Geometry: final body of the model. Coordinates: model frame, mm. A direction names the side the tool comes from. Round coordinates to 2 decimals unless told otherwise and drop trailing zeros. Loops run counter-clockwise (first coordinate to the right, second up) from the corner with the lowest first, then second, coordinate; pieces in that order, holes last. Notation, with made-up numbers: (54.25, 69) - (97.25, 69) arc R16 cw to (97.25, 99) - close; hole circle Ø5 at (-10, 40.25). An arc over 180 degrees is marked (long way). Answer as CSV lines item,"result".
from build123d import *

# Parameters (mm, degrees)
F0_R     = 1.5
F2_DEPTH = 35
F1_R     = 3
F3_DEPTH = 2.52
F4_R     = 1


with BuildPart() as f2:
    # F0 (on Top) → F2 (new body)
    with BuildSketch(Plane.XY):
        Circle(F0_R)
    extrude(amount=-F2_DEPTH)

    # F1 (on Top) → F3 (join)
    with BuildSketch(Plane.XY):
        Circle(F1_R)
    extrude(amount=F3_DEPTH)

    # F4
    f4_edges = [f2.edges().sort_by_distance(p)[0] for p in [
        (-3, 0, 2.52),
    ]]
    fillet(f4_edges, radius=F4_R)


solid = f2.part
(1) Access query for faces 1 (the face through (1.3, -1.3, 0)), 2 (the face through (0, 0, 2.52)). Directions: +Z, -Z, +X, -X, +Y, -Y. A direction counts if a zero-diameter tool reaches every point of the face in a straight line with its end or side. Return the directions, or none.
Findings below:
face 1,"-Z"
face 2,"+Z, +X, -X, +Y, -Y"
(2) Section A-A (x = 0). Output: boundary loops of the cut face in (y, z), and give its area (3 significant figures).
Findings below:
outline,"(-3, 0) - (-1.5, 0) - (-1.5, -35) - (1.5, -35) - (1.5, 0) - (3, 0) - (3, 1.52) arc R1 ccw to (2, 2.52) - (-2, 2.52) arc R1 ccw to (-3, 1.52) - close"
area,"120 mm2"
(3) Pin query (flat end, axial travel): P1, Ø1.5, axis at y = -2, z = -12.5, coming from the +X side; P2, Ø3, axis at y = -1, z = -13, coming from the -X side; P3, Ø1.5, axis at x = -2, z = -13.5, coming from the -Y side. Return the tip coordinate at first contact, or that it passes through.
Findings below:
P1,"x = 0.83"
P2,"x = -1.5"
P3,"y = -0.83"
(4) Section C-C (z = -26). Output: boundary loops of the cut face in (x, y), and give its area (3 significant figures).
Findings below:
outline,"circle Ø3 at (0, 0)"
area,"7.07 mm2"
(5) Material intervals for line 1 along Z through (x, y) = (0.7, -1.5); line 2 along Z through (x, y) = (2.6, 0.75); line 3 along Y through (x, z) = (0.65, -13), sorted ascending.
Findings below:
line 1,"0 to 2.52"
line 2,"0 to 2.23"
line 3,"-1.35 to 1.35"
